Can you work these out from the model? Positions are in its coordinate system, mm. Face numbers are marked on the shaded views. A direction names the side the tool comes from. Coordinates: 2 decimals unless noted, no trailing zeros. Loops run counter-clockwise (first coordinate to the right, second up) from the corner with the lowest first, then second, coordinate; pieces in that order, holes last. Notation, with made-up numbers: M -24,-18.5 L -2,-18.5 A18 ccw -2,1.5 Z; hole C 8.5,-18.75 d6. An arc over 180 degrees is marked long. Answer as a JSON object with one key per item and string values. Group by question number.
Item 1: Suppose I cut it at D-D (z = 448). Write out the boundary of the cut face in (x, y), then the cut area to 3 significant figures.
Item 2: Suppose I cut it at B-B (y = 11.75). Write out the boundary of the cut face in (x, z).
Item 3: Suppose I cut it at C-C (y = 23.5). Write out the boundary of the cut face in (x, z).
Item 4: Which directions (+Z, -Z, +X, -X, +Y, -Y) give clear straight access to the entire face, cutting with the end or side of a thin tool? Please do the marked faces 5 and 6.
Item 5: We'd pull the mould along Z, two halves only. Please class the marked faces 1, 2, 3 and 4: +Z half, -Z half, draft (parallel to the pull), parting line (faces both ways), or undercut.
Item 6: If I drill on line 1 (Z direction, x = -314.5, y = 8.5); line 2 (X direction, y = 25.5, z = 450), over which ranges is the centre line in solid material (lowest first)?
Item 7: I'm going to push a flat-ended pin straight in: pin 1 Ø8 at (y, z) = (11, 401) entering from +X. Where does the tip first touch, or does it pass through?
Item 8: Suppose I cut it at A-A (x = -323.5). Write out the boundary of the cut face in (y, z).
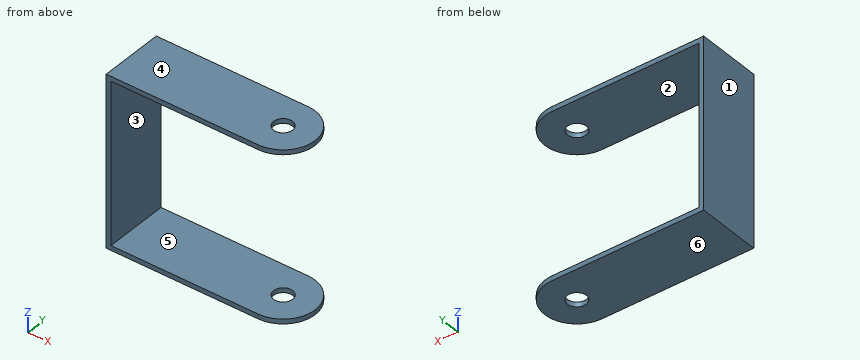
```python
from build123d import *

# Parameters (mm, degrees)
SKETCH1_W           = 77.5
SKETCH1_H           = 72
BOSS_EXTRUDE2_DEPTH = 27
SKETCH2_W           = 73.5
SKETCH2_H           = 68
CUT_EXTRUDE1_DEPTH  = 27
SKETCH7_W           = 2
SKETCH7_H           = 68
CUT_EXTRUDE2_DEPTH  = 27
FILLET6_R           = 13.5
FILLET7_R           = 13.5
SKETCH9_R           = 4
CUT_EXTRUDE3_DEPTH  = 94


with BuildPart() as part:
    # Sketch1 → Boss-Extrude2 (new body)
    with BuildSketch(Plane(origin=(0, 0, 0), x_dir=(1, 0, 0), z_dir=(0, 1, 0))):
        with Locations((-311.893899893, -425.385906876)):
            Rectangle(SKETCH1_W, SKETCH1_H)
    extrude(amount=BOSS_EXTRUDE2_DEPTH)

    # Sketch2 → Cut-Extrude1 (cut)
    with BuildSketch(Plane(origin=(0, 27, 0), x_dir=(1, 0, 0), z_dir=(0, 1, 0))):
        with Locations((-311.893899893, -425.385906876)):
            Rectangle(SKETCH2_W, SKETCH2_H)
    extrude(amount=-CUT_EXTRUDE1_DEPTH, mode=Mode.SUBTRACT)

    # Sketch7 → Cut-Extrude2 (cut)
    with BuildSketch(Plane(origin=(0, 27, 0), x_dir=(1, 0, 0), z_dir=(0, 1, 0))):
        with Locations((-274.143899893, -425.385906876)):
            Rectangle(SKETCH7_W, SKETCH7_H)
    extrude(amount=-CUT_EXTRUDE2_DEPTH, mode=Mode.SUBTRACT)

    # Fillet6
    fillet6_edges = [part.edges().sort_by_distance(p)[0] for p in [
        (-273.143899893, 0, 460.385906876),
        (-273.143899893, 27, 460.385906876),
    ]]
    fillet(fillet6_edges, radius=FILLET6_R - 0.0001)  # a hair under: the kernel refuses the full size

    # Fillet7
    fillet7_edges = [part.edges().sort_by_distance(p)[0] for p in [
        (-273.143899893, 0, 390.385906876),
        (-273.143899893, 27, 390.385906876),
    ]]
    fillet(fillet7_edges, radius=FILLET7_R - 0.0001)  # a hair under: the kernel refuses the full size

    # Sketch9 → Cut-Extrude3 (cut)
    with BuildSketch(Plane.XY.offset(461.385906876)):
        with Locations((-286.643899893, 13.5)):
            Circle(SKETCH9_R)
    extrude(amount=-CUT_EXTRUDE3_DEPTH, mode=Mode.SUBTRACT)


solid = part.part
```
From the geometry:
{
 "1": {"outline": "M -350.64,0 L -348.64,0 L -348.64,27 L -350.64,27 Z", "area": "54.0 mm2"},
 "2": {"outline": "M -350.64,389.39 L -290.24,389.39 L -290.24,391.39 L -348.64,391.39 L -348.64,459.39 L -290.24,459.39 L -290.24,461.39 L -350.64,461.39 Z; M -283.05,389.39 L -273.26,389.39 L -273.26,391.39 L -283.05,391.39 Z; M -283.05,459.39 L -273.26,459.39 L -273.26,461.39 L -283.05,461.39 Z"},
 "3": {"outline": "M -350.64,389.39 L -277.57,389.39 L -277.57,391.39 L -348.64,391.39 L -348.64,459.39 L -277.57,459.39 L -277.57,461.39 L -350.64,461.39 Z"},
 "4": {"face 5": "+X, +Y, -Y", "face 6": "-Z, +X, -X, +Y, -Y"},
 "5": {"face 1": "draft", "face 2": "undercut", "face 3": "undercut", "face 4": "+Z half"},
 "6": {"line 1": "389.39 to 391.39, 459.39 to 461.39", "line 2": "-350.64 to -348.64"},
 "7": {"pin 1": "x = -348.64"},
 "8": {"outline": "M 0,389.39 L 27,389.39 L 27,391.39 L 0,391.39 Z; M 0,459.39 L 27,459.39 L 27,461.39 L 0,461.39 Z"}
}
